Can you work these out from the model? Positions are in its coordinate system, mm. Give positions to 0.01 mm unless a question says otherwise; leave off trailing zeros. Loops run counter-clockwise (first coordinate to the right, second up) from the corner with the lowest first, then second, coordinate; pieces in that order, holes last. Notation, with made-up numbers: (-25.5, -17) - (29.5, -17) arc R10 ccw to (29.5, -4) - close; hole circle Ø4 at (16.5, 50.5). An arc over 180 degrees is marked (long way). Answer as a JSON object with one key per item and string values. Group by question number.
Item 1: Suppose I cut it at D-D on y = -15.5. Write out the boundary of the cut face in (x, z), and give its area (3 significant figures).
Item 2: Will these pins go through, and if not, where does the flat tip stop? pin 1 (4 mm diameter, centred on x = 50.5, y = 29, fed in from +Z); pin 2 (1.5 mm diameter, centred on y = -35.5, z = -28, fed in from -X); pin 3 (1 mm diameter, centred on x = 13, z = 15, fed in from -Y); pin 4 (1.5 mm diameter, centred on y = -16.5, z = -11.5, fed in from -X).
Item 3: Suppose I cut it at A-A on y = -4. Write out the boundary of the cut face in (x, z).
Item 4: Suppose I cut it at C-C on z = 1.5. Write out the boundary of the cut face in (x, y), and give its area (3 significant figures).
Item 5: Thinking about a two-plate mould opening in X: for faces 1 (the flat face through (32, 0, -37.155)), 2 (the cylindrical face through (47.373, 13.363, -0.52)), 3 (the cylindrical face through (6.11, -39.154, 0.236)), which applies, pulls with the +X half, pulls with the -X half, needs draft (parallel to the pull), parting line crosses it, or undercut?
Item 6: Please list where these lines run through material, in increasing order: L1, parallel to Z at x = 30, y = 0; L2, parallel to Y at x = 35, z = 0; L3, parallel to Y at x = 45, z = 5.
Item 7: Suppose I cut it at B-B on x = 38. Write out the boundary of the cut face in (y, z), and give its area (3 significant figures).
from build123d import *

# Parameters (mm, degrees)
F0_W     = 89.89758
F0_H     = 74.309834
F1_DEPTH = 82.804
F2_R     = 20.32
F4_D     = 25.4
F6_D     = 25.4


with BuildPart() as f1:
    # F0 (on Right) → F1 (new body)
    with BuildSketch(Plane.YZ):
        Rectangle(F0_W, F0_H)
    extrude(amount=F1_DEPTH)

    # F2
    f2_edges = [f1.edges().sort_by_distance(p)[0] for p in [
        (41.402, 44.94879, 37.154917),
        (41.402, -44.94879, 37.154917),
        (0, 0, 37.154917),
        (82.804, 0, 37.154917),
        (82.804, 0, -37.154917),
        (82.804, 44.94879, 0),
        (82.804, -44.94879, 0),
        (41.402, -44.94879, -37.154917),
        (0, -44.94879, 0),
        (41.402, 44.94879, -37.154917),
        (0, 44.94879, 0),
        (0, 0, -37.154917),
    ]]
    fillet(f2_edges, radius=F2_R)

    # F4 (through all)
    with Locations(Plane.XY.offset(37.154917)):
        with Locations((45.72, 0.77121)):
            Hole(F4_D / 2)

    # F6 (through all)
    with Locations(Plane.YZ.offset(82.804)):
        with Locations((0, 0)):
            Hole(F6_D / 2)


solid = f1.part
Worked out:
{
 "1": {"outline": "(0, -16.83) arc R20.32 ccw to (20.32, -37.15) - (62.48, -37.15) arc R20.32 ccw to (82.8, -16.83) - (82.8, 16.83) arc R20.32 ccw to (62.48, 37.15) - (20.32, 37.15) arc R20.32 ccw to (0, 16.83) - close", "area": "5,800 mm2"},
 "2": {"pin 1": "stops at z = 37.02", "pin 2": "stops at x = 6.43", "pin 3": "stops at y = -43.77", "pin 4": "stops at x = 0"},
 "3": {"outline": "(0, -16.83) arc R20.32 ccw to (20.32, -37.15) - (33.95, -37.15) - (33.95, -12.05) - (0, -12.05) - close; (0, 12.05) - (33.95, 12.05) - (33.95, 37.15) - (20.32, 37.15) arc R20.32 ccw to (0, 16.83) - close; (57.49, -37.15) - (62.48, -37.15) arc R20.32 ccw to (82.8, -16.83) - (82.8, -12.05) - (57.49, -12.05) - close; (57.49, 12.05) - (82.8, 12.05) - (82.8, 16.83) arc R20.32 ccw to (62.48, 37.15) - (57.49, 37.15) - close"},
 "4": {"outline": "(0, -24.63) arc R20.32 ccw to (20.32, -44.95) - (62.48, -44.95) arc R20.32 ccw to (82.8, -24.63) - (82.8, -12.61) - (0, -12.61) - close; (0, 12.61) - (41.13, 12.61) arc R12.7 cw to (50.31, 12.61) - (82.8, 12.61) - (82.8, 24.63) arc R20.32 ccw to (62.48, 44.95) - (20.32, 44.95) arc R20.32 ccw to (0, 24.63) - close", "area": "5,000 mm2"},
 "5": {"face 1": "needs draft", "face 2": "undercut", "face 3": "pulls with the -X half"},
 "6": {"L1": "z = -37.15 to -12.7, 12.7 to 37.15", "L2": "y = -44.95 to -12.7, 12.7 to 44.95", "L3": "y = -44.95 to -11.91, 13.45 to 44.95"},
 "7": {"outline": "(-44.95, -16.83) arc R20.32 ccw to (-24.63, -37.15) - (-9.31, -37.15) - (-9.31, -8.63) arc R12.7 cw to (-9.31, 8.63) - (-9.31, 37.15) - (-24.63, 37.15) arc R20.32 ccw to (-44.95, 16.83) - close; (10.86, -37.15) - (24.63, -37.15) arc R20.32 ccw to (44.95, -16.83) - (44.95, 16.83) arc R20.32 ccw to (24.63, 37.15) - (10.86, 37.15) - (10.86, 6.59) arc R12.7 cw to (10.86, -6.59) - close", "area": "4,770 mm2"}
}
